The drawing under review shows one solid part. Ordinate dimensions are in mm from its lowest x, y, z. Coordinates: 2 decimals unless noted, no trailing zeros. Order: outer loops, then holes, each group sorted by start corner. A loop starts at its lowest first (then second) coordinate and runs counter-clockwise, first axis right, second up. Notation, with made-up numbers: M 36,62 L 88,62 A22 cw 88,87 Z; hole C 56.25,49.5 d1. An arc over 180 degrees is marked long. Answer as a JSON object with one key per item and string values.
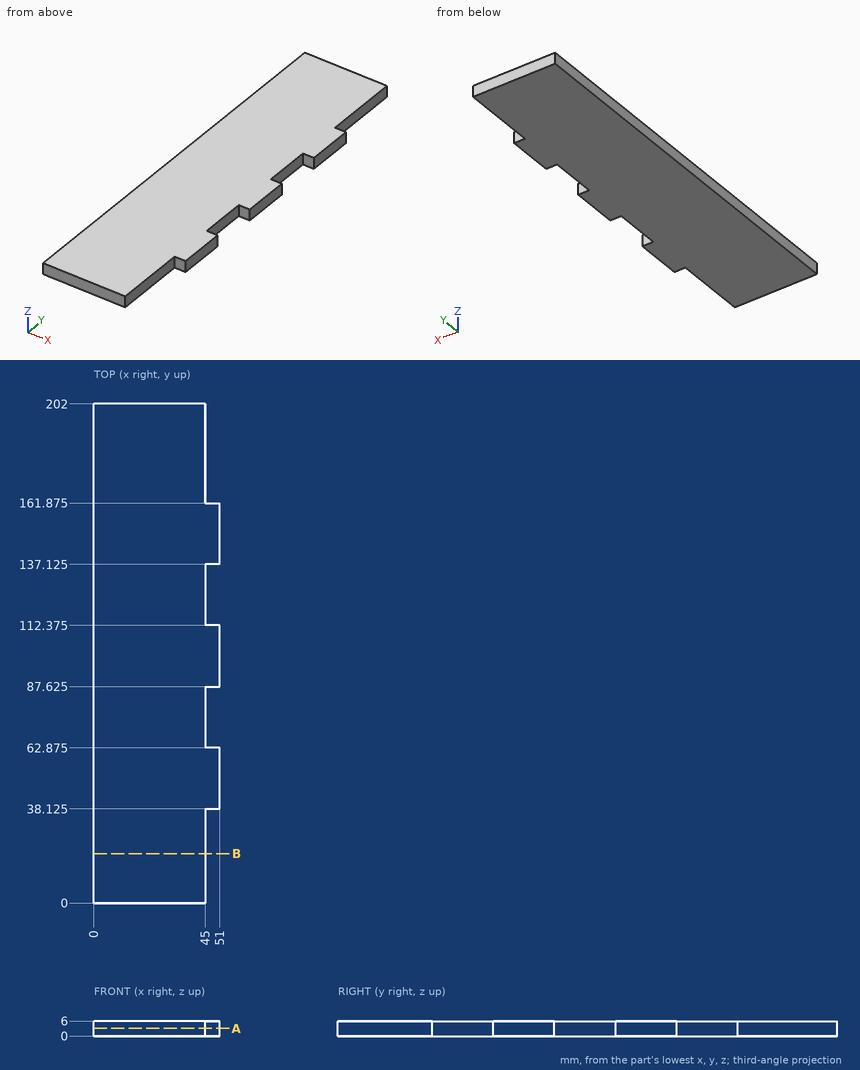
1) To check wall thickness, follow L1, parallel to Y at x = 47.5, z = 4.1 (3 decimals); L2, parallel to X at y = 118, z = 5.7. State the ranges of each line that lie inside material, in increasing order.
Taken from the geometry:
{"L1": "y = 38.125 to 62.875, 87.625 to 112.375, 137.125 to 161.875", "L2": "x = 0 to 45"}
2) Add section B-B (y = 20). State the section outline as (x, z) points, and give its area (3 significant figures).
Taken from the geometry:
{"outline": "M 0,0 L 45,0 L 45,6 L 0,6 Z", "area": "270 mm2"}
3) Add section A-A (z = 3.1). State the section outline as (x, y) points (3 decimals).
Taken from the geometry:
{"outline": "M 0,0 L 45,0 L 45,38.125 L 51,38.125 L 51,62.875 L 45,62.875 L 45,87.625 L 51,87.625 L 51,112.375 L 45,112.375 L 45,137.125 L 51,137.125 L 51,161.875 L 45,161.875 L 45,202 L 0,202 Z"}
4) Insertion check: pin 1 Ø1.8 at (y, z) = (129.5, 1.5) entering from +X; pin 2 Ø3 at (x, z) = (47, 2) entering from +Y (3 decimals); pin 3 Ø3 at (x, z) = (48.5, 3.5) entering from -Y (3 decimals). Each pin has a flat end and moves straight along its axis. Give the tip position at first contact, or say it passes through.
Taken from the geometry:
{"pin 1": "stops at x = 45", "pin 2": "stops at y = 161.875", "pin 3": "stops at y = 38.125"}
